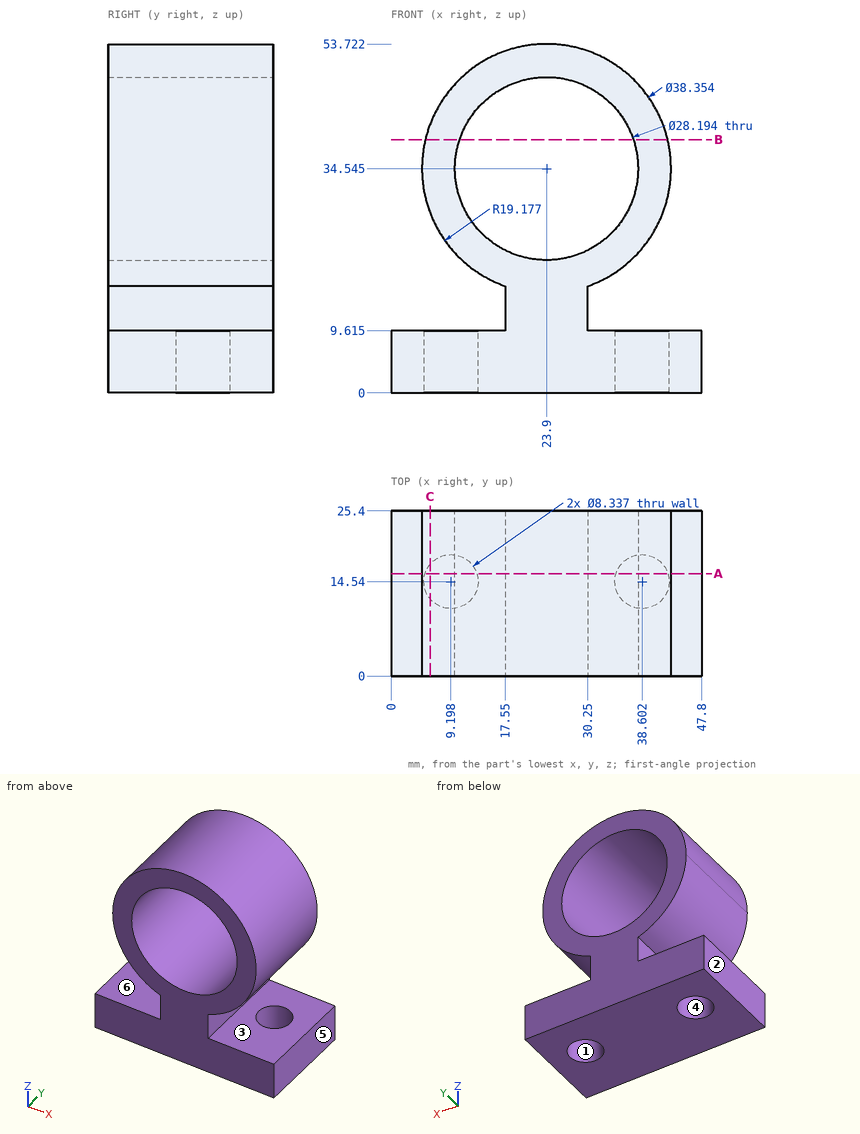
Verification items for this drawing (mm, ordinates from the low corner). A direction names the side the tool comes from. Give positions to 0.01 mm unless a question says otherwise; leave off trailing zeros. Loops run counter-clockwise (first coordinate to the right, second up) from the corner with the lowest first, then second, coordinate; pieces in that order, holes last. Notation, with made-up numbers: M 60.5,-9.75 L 72.5,-9.75 A10 ccw 72.5,6.25 Z; hole C 34,38 d9. An arc over 180 degrees is marked long. Answer as a JSON object with one key per item and string values. Group by question number.
Q1. Go/stop test with flat-tipped pins: P1, Ø12, axis at x = 38.5, y = 7.5, coming from the +Z side (1 decimal); P2, Ø2, axis at x = 28, y = 6.5, coming from the +Z side; P3, Ø3, axis at x = 18, y = 12.5, coming from the +Z side. Record where each tip stops, or that it passes through.
Q2. Access from +Z, -Z, +X, -X, +Y, -Y to the whole of each face (thin tool, end or side, straight path). Record for the marked faces 4, 5 and 6.
Q3. Release check for a two-part mould opening along X. For the marked faces 1, 2 and 3 record: released by +X, released by -X, zero draft, split by the parting line, or undercut.
Q4. Cross-section at B-B on z = 39. Record the cut outline in (x, y) (1 decimal).
Q5. Material ranges on line 1 along Z through (x, y) = (32, 7.75) (1 decimal); line 2 along Z through (x, y) = (4, 17.5) (1 decimal); line 3 along Z through (x, y) = (35.5, 6) (1 decimal), recorded low to high. Write a range as [from, to].
Q6. Cross-section at A-A on y = 15.75. Give the number of separate pieces and of enclosed holes in the cut face, then the cut area to 3 significant figures.
Q7. Cross-section at C-C on x = 6. Record the cut outline in (y, z) (1 decimal), then the cut area to 3 significant figures.
Evaluation:
{
 "1": {"P1": "stops at z = 51.7", "P2": "stops at z = 53.47", "P3": "stops at z = 53.21"},
 "2": {"face 4": "-Z", "face 5": "+Z, -Z, +X, +Y, -Y", "face 6": "-X, +Y, -Y"},
 "3": {"face 1": "undercut", "face 2": "released by -X", "face 3": "zero draft"},
 "4": {"outline": "M 5.2,0 L 10.5,0 L 10.5,25.4 L 5.2,25.4 Z; M 37.3,0 L 42.6,0 L 42.6,25.4 L 37.3,25.4 Z"},
 "5": {"line 1": "z = [0, 9.6], [17.2, 23], [46.1, 51.9]", "line 2": "z = [0, 9.6]", "line 3": "z = [0, 9.6], [19.3, 26.5], [42.6, 49.8]"},
 "6": {"separate pieces": "3", "enclosed holes": "1", "area": "915 mm2"},
 "7": {"outline": "M 0,0 L 11.9,0 L 11.9,9.6 L 0,9.6 Z; M 0,27.7 L 25.4,27.7 L 25.4,41.4 L 0,41.4 Z; M 17.2,0 L 25.4,0 L 25.4,9.6 L 17.2,9.6 Z", "area": "542 mm2"}
}
